```python
from build123d import *

# Parameters (mm, degrees)
SKETCH_2_W          = 28
SKETCH_2_H          = 12
EXTRUDE_1_DEPTH     = 9.5
SKETCH_3_W          = 31.5
SKETCH_3_H          = 12.3
EXTRUDE_2_DEPTH     = 1
SKETCH_4_W          = 35
SKETCH_4_H          = 18
SKETCH_4_R          = 1.15
SKETCH_4_R_2        = 0.4
EXTRUDE_3_DEPTH     = 1.6
SKETCH_6_R          = 3.5
CUT_EXTRUDE_1_DEPTH = 2


with BuildPart() as part:
    # 草图2 → 凸台-拉伸1 (new body)
    with BuildSketch(Plane.XY):
        Rectangle(SKETCH_2_W, SKETCH_2_H)
    extrude(amount=EXTRUDE_1_DEPTH)

    # 草图3 → 凸台-拉伸2 (add)
    with BuildSketch(Plane(origin=(0, 0, 0), x_dir=(-1, 0, 0), z_dir=(0, 0, -1))):
        Rectangle(SKETCH_3_W, SKETCH_3_H)
    extrude(amount=EXTRUDE_2_DEPTH)

    # 草图4 → 凸台-拉伸3 (add)
    with BuildSketch(Plane.XZ.offset(6)):
        with Locations((-1.7, 0.5)):
            Rectangle(SKETCH_4_W, SKETCH_4_H)
        with Locations(Location((-16.7, 6.85, 0), (0, 0, 270))):
            Circle(SKETCH_4_R, mode=Mode.SUBTRACT)
        with Locations(Location((14.8, -7.5, 0), (0, 0, 270))):
            Circle(SKETCH_4_R_2, mode=Mode.SUBTRACT)
        with Locations(Location((12.26, -7.5, 0), (0, 0, 270))):
            Circle(SKETCH_4_R_2, mode=Mode.SUBTRACT)
        with Locations(Location((9.72, -7.5, 0), (0, 0, 270))):
            Circle(SKETCH_4_R_2, mode=Mode.SUBTRACT)
        with Locations(Location((7.18, -7.5, 0), (0, 0, 270))):
            Circle(SKETCH_4_R_2, mode=Mode.SUBTRACT)
        with Locations(Location((4.64, -7.5, 0), (0, 0, 270))):
            Circle(SKETCH_4_R_2, mode=Mode.SUBTRACT)
    extrude(amount=EXTRUDE_3_DEPTH)

    # 草图6 → 切除-拉伸1 (cut)
    with BuildSketch(Plane.XY.offset(9.5)):
        Circle(SKETCH_6_R)
    extrude(amount=-CUT_EXTRUDE_1_DEPTH, mode=Mode.SUBTRACT)


solid = part.part
```
Here's how the part is built. I have some questions about the finished solid (model axes, mm). A direction names the side the tool comes from. Coordinates: 2 decimals unless noted, no trailing zeros. Loops run counter-clockwise (first coordinate to the right, second up) from the corner with the lowest first, then second, coordinate; pieces in that order, holes last. Notation, with made-up numbers: M 29.25,-40 L 72.25,-40 A17 ccw 72.25,-29 Z; hole C -24,47.25 d11. An arc over 180 degrees is marked long. One line per item, written item: value.
1. Thinking about a two-plate mould opening in Y: for faces 6 (the flat face through (0, 6, 5)), 7 (the cylindrical face through (3.233, -1.341, 8.514)), 8 (the flat face through (0, 0, 7.5)), 9 (the cylindrical face through (15.197, -6.789, -7.448)), which applies, +Y half, -Y half, draft (parallel to the pull), parting line (faces both ways), or undercut?
Geometry says:
face 6: +Y half
face 7: undercut
face 8: undercut
face 9: draft
2. Please list where these lines run through material, in increasing order: probe 1 along X at (y, z) = (-6.4, -7.5); probe 2 along X at (y, z) = (0, -0.25); probe 3 along X at (y, z) = (1.5, 3.75).
Geometry says:
probe 1: x = -19.2 to 4.24, 5.04 to 6.78, 7.58 to 9.32, 10.12 to 11.86, 12.66 to 14.4, 15.2 to 15.8
probe 2: x = -15.75 to 15.75
probe 3: x = -14 to 14
3. Imagine slicing it at C-C (z = -7.5). List the corners of the cut face in (x, y) for me, and give its area (3 significant figures).
Geometry says:
outline: M -19.2,-7.6 L 4.24,-7.6 L 4.24,-6 L -19.2,-6 Z; M 5.04,-7.6 L 6.78,-7.6 L 6.78,-6 L 5.04,-6 Z; M 7.58,-7.6 L 9.32,-7.6 L 9.32,-6 L 7.58,-6 Z; M 10.12,-7.6 L 11.86,-7.6 L 11.86,-6 L 10.12,-6 Z; M 12.66,-7.6 L 14.4,-7.6 L 14.4,-6 L 12.66,-6 Z; M 15.2,-7.6 L 15.8,-7.6 L 15.8,-6 L 15.2,-6 Z
area: 49.6 mm2
4. Imagine slicing it at B-B (x = 12.26). List the corners of the cut face in (y, z) for me, and give its area (3 significant figures).
Geometry says:
outline: M -7.6,-8.5 L -6,-8.5 L -6,-7.9 L -7.6,-7.9 Z; M -7.6,-7.1 L -6,-7.1 L -6,-1 L 6.15,-1 L 6.15,0 L 6,0 L 6,9.5 L -7.6,9.5 Z
area: 154 mm2
5. Will these pins go through, and if not, where does the flat tip stop? pin 1 Ø0.5 at (y, z) = (-2.5, -0.5) entering from +X; pin 2 Ø4 at (x, y) = (0, 0) entering from +Z; pin 3 Ø5 at (y, z) = (3, 4.5) entering from +X.
Geometry says:
pin 1: stops at x = 15.75
pin 2: stops at z = 7.5
pin 3: stops at x = 14
6. Imagine slicing it at D-D (x = 0). List the corners of the cut face in (y, z) for me.
Geometry says:
outline: M -7.6,-8.5 L -6,-8.5 L -6,-1 L 6.15,-1 L 6.15,0 L 6,0 L 6,9.5 L 3.5,9.5 L 3.5,7.5 L -3.5,7.5 L -3.5,9.5 L -7.6,9.5 Z
7. On a 3-axis mill with a long thin cutter (end or side, diameter ignored), from which of +Z, -Z, +X, -X, +Y, -Y can I reach the whole of each face in a straight line? I mean faces 1 (the flat face through (-15.75, 0, -0.5)), 2 (the flat face through (-2, -7, -8.5)), 3 (the flat face through (0, 0, -1)), 4 (the flat face through (14, 0, 5)), 5 (the flat face through (15.75, 0, -0.5)). Say none if no direction works.
Geometry says:
face 1: +Z, -Z, -X, +Y
face 2: -Z, +X, -X, +Y, -Y
face 3: -Z, +X, -X, +Y
face 4: +Z, +X, +Y
face 5: +Z, -Z, +X, +Y
8. Imagine slicing it at A-A (z = 6.85). List the corners of the cut face in (x, y) for me.
Geometry says:
outline: M -19.2,-7.6 L -17.85,-7.6 L -17.85,-6 L -19.2,-6 Z; M -15.55,-7.6 L 15.8,-7.6 L 15.8,-6 L 14,-6 L 14,6 L -14,6 L -14,-6 L -15.55,-6 Z
